CAD build for the part. Positions are in the model's coordinates, mm. Face numbers are marked on the shaded views. Round coordinates to 2 decimals unless told otherwise and drop trailing zeros. Order: outer loops, then holes, each group sorted by start corner. A loop starts at its lowest first (then second) coordinate and runs counter-clockwise, first axis right, second up. Notation, with made-up numbers: M 74.25,12 L 124.25,12 A26 cw 124.25,27 Z; hole C 29.5,67.5 d3. An arc over 180 degrees is marked long. Put each result on its own line as item: value.
```python
from build123d import *

# Parameters (mm, degrees)
SKETCH1_R           = 6
SKETCH1_R_2         = 3
BOSS_EXTRUDE1_DEPTH = 3
SKETCH3_R           = 3
BOSS_EXTRUDE3_DEPTH = 3
SKETCH4_R           = 8
SKETCH4_R_2         = 3
BOSS_EXTRUDE4_DEPTH = 12
SKETCH6_R           = 8
SKETCH6_R_2         = 3
BOSS_EXTRUDE5_DEPTH = 12


with BuildPart() as part:
    # Sketch1 → Boss-Extrude1 (new body)
    # profile 1 of 4: a face of its own
    with BuildSketch(Plane(origin=(0, 0, 0), x_dir=(1, 0, 0), z_dir=(0, 1, 0))):
        with BuildLine():
            ThreePointArc((42.894958583, -3.003752345), (43.557934635, -6.502479184), (45.856433127, -9.222319513))
            ThreePointArc((45.856433127, -9.222319513), (50.229473419, -29), (30.914979544, -35.101676259))
            ThreePointArc((30.914979544, -35.101676259), (27.410279478, -34.471038339), (24.048805129, -35.646247655))
            ThreePointArc((24.048805129, -35.646247655), (0, -43), (-24.048805129, -35.646247655))
            ThreePointArc((-24.048805129, -35.646247655), (-27.410279478, -34.471038339), (-30.914979544, -35.101676259))
            ThreePointArc((-30.914979544, -35.101676259), (-50.229473419, -29), (-45.856433127, -9.222319513))
            ThreePointArc((-45.856433127, -9.222319513), (-43.557934635, -6.502479184), (-42.894958583, -3.003752345))
            ThreePointArc((-42.894958583, -3.003752345), (-37.239092363, 21.5), (-18.846153454, 38.65))
            ThreePointArc((-18.846153454, 38.65), (-16.147655157, 40.973517523), (-14.941453584, 44.323995772))
            ThreePointArc((-14.941453584, 44.323995772), (0, 58), (14.941453584, 44.323995772))
            ThreePointArc((14.941453584, 44.323995772), (16.147655157, 40.973517523), (18.846153454, 38.65))
            ThreePointArc((18.846153454, 38.65), (37.239092363, 21.5), (42.894958583, -3.003752345))
        make_face()
        with Locations((37.239092363, -21.5)):
            Circle(SKETCH1_R, mode=Mode.SUBTRACT)
        with Locations((-37.239092363, -21.5)):
            Circle(SKETCH1_R, mode=Mode.SUBTRACT)
        with Locations((0, 43)):
            Circle(SKETCH1_R, mode=Mode.SUBTRACT)
    # profile 2 of 4: a face of its own
    with BuildSketch(Plane(origin=(0, 0, 0), x_dir=(1, 0, 0), z_dir=(0, 1, 0))):
        with Locations((-37.239092363, -21.5)):
            Circle(SKETCH1_R)
        with Locations(Location((-37.239092363, -21.5, 0), (0, 0, 270))):
            Circle(SKETCH1_R_2, mode=Mode.SUBTRACT)
    # profile 3 of 4: a face of its own
    with BuildSketch(Plane(origin=(0, 0, 0), x_dir=(1, 0, 0), z_dir=(0, 1, 0))):
        with Locations((37.239092363, -21.5)):
            Circle(SKETCH1_R)
        with Locations(Location((37.239092363, -21.5, 0), (0, 0, 270))):
            Circle(SKETCH1_R_2, mode=Mode.SUBTRACT)
    # profile 4 of 4: a face of its own
    with BuildSketch(Plane(origin=(0, 0, 0), x_dir=(1, 0, 0), z_dir=(0, 1, 0))):
        with Locations((0, 43)):
            Circle(SKETCH1_R)
        with Locations(Location((0, 43, 0), (0, 0, 270))):
            Circle(SKETCH1_R_2, mode=Mode.SUBTRACT)
    extrude(amount=BOSS_EXTRUDE1_DEPTH)

    # Sketch3 → Boss-Extrude3 (add)
    with BuildSketch(Plane(origin=(0, 3, 0), x_dir=(1, 0, 0), z_dir=(0, 1, 0))):
        with BuildLine():
            ThreePointArc((13.496951609, 40.286875), (0, 53.5), (-13.496951609, 40.286875))
            ThreePointArc((-13.496951609, 40.286875), (-14.175747319, 38.14126951), (-15.905498529, 36.701704545))
            ThreePointArc((-15.905498529, 36.701704545), (-34.641016151, 20), (-39.737357763, -4.576286487))
            ThreePointArc((-39.737357763, -4.576286487), (-40.119181988, -6.794077459), (-41.637932994, -8.454734533))
            ThreePointArc((-41.637932994, -8.454734533), (-46.332359102, -26.75), (-28.140981385, -31.832140467))
            ThreePointArc((-28.140981385, -31.832140467), (-25.943434669, -31.347192051), (-23.831859234, -32.125418059))
            ThreePointArc((-23.831859234, -32.125418059), (0, -40), (23.831859234, -32.125418059))
            ThreePointArc((23.831859234, -32.125418059), (25.943434669, -31.347192051), (28.140981385, -31.832140467))
            ThreePointArc((28.140981385, -31.832140467), (46.332359102, -26.75), (41.637932994, -8.454734533))
            ThreePointArc((41.637932994, -8.454734533), (40.119181988, -6.794077459), (39.737357763, -4.576286487))
            ThreePointArc((39.737357763, -4.576286487), (34.641016151, 20), (15.905498529, 36.701704545))
            ThreePointArc((15.905498529, 36.701704545), (14.175747319, 38.14126951), (13.496951609, 40.286875))
        make_face()
        with Locations(Location((0, 43, 0), (0, 0, 270))):
            Circle(SKETCH3_R, mode=Mode.SUBTRACT)
        with Locations(Location((-37.239092363, -21.5, 0), (0, 0, 270))):
            Circle(SKETCH3_R, mode=Mode.SUBTRACT)
        with Locations(Location((37.239092363, -21.5, 0), (0, 0, 270))):
            Circle(SKETCH3_R, mode=Mode.SUBTRACT)
    extrude(amount=BOSS_EXTRUDE3_DEPTH)

    # Sketch4 → Boss-Extrude4 (add)
    with BuildSketch(Plane(origin=(0, 6, 0), x_dir=(1, 0, 0), z_dir=(0, 1, 0))):
        with Locations(Location((0, 43, 0), (0, 0, 270))):
            Circle(SKETCH4_R)
        with Locations(Location((0, 43, 0), (0, 0, 270))):
            Circle(SKETCH4_R_2, mode=Mode.SUBTRACT)
    extrude(amount=BOSS_EXTRUDE4_DEPTH)

    # Sketch6 → Boss-Extrude5 (add)
    # profile 1 of 2: a face of its own
    with BuildSketch(Plane(origin=(0, 6, 0), x_dir=(1, 0, 0), z_dir=(0, 1, 0))):
        with Locations(Location((-37.239092363, -21.5, 0), (0, 0, 270))):
            Circle(SKETCH6_R)
        with Locations(Location((-37.239092363, -21.5, 0), (0, 0, 270))):
            Circle(SKETCH6_R_2, mode=Mode.SUBTRACT)
    # profile 2 of 2: a face of its own
    with BuildSketch(Plane(origin=(0, 6, 0), x_dir=(1, 0, 0), z_dir=(0, 1, 0))):
        with Locations(Location((37.239092363, -21.5, 0), (0, 0, 270))):
            Circle(SKETCH6_R)
        with Locations(Location((37.239092363, -21.5, 0), (0, 0, 270))):
            Circle(SKETCH6_R_2, mode=Mode.SUBTRACT)
    extrude(amount=BOSS_EXTRUDE5_DEPTH)


solid = part.part
```
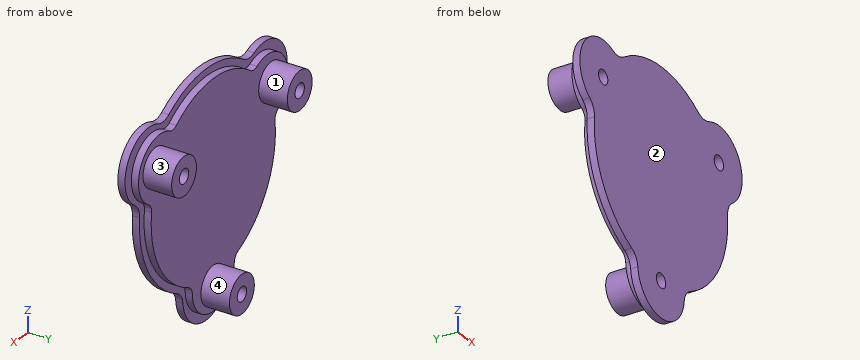
Item 1: Mould opens along X. For the marked faces 1, 2, 3 and 4 say: pulls with the +X half, pulls with the -X half, needs draft (parallel to the pull), parting line crosses it, or undercut.
Answers below:
face 1: undercut
face 2: needs draft
face 3: undercut
face 4: parting line crosses it
Item 2: Probe line 1 along X through (y, z) = (11, 21.5); line 2 along X through (y, z) = (12.75, -43); line 3 along X through (y, z) = (11.5, 19.5). List the from-to ranges inside material, lowest first. Write a range as [from, to].
Answers below:
line 1: [-45.24, -40.24], [-34.24, -29.24], [29.24, 34.24], [40.24, 45.24]
line 2: [-8, -3], [3, 8]
line 3: [-44.99, -39.48], [-35, -29.49], [29.49, 35], [39.48, 44.99]
Item 3: Pin check, flat tips, straight feed: P1, Ø10, axis at x = 36.5, y = 16, coming from the +Z side; P2, Ø12, axis at x = 15.5, z = -25, coming from the +Y side; P3, Ø8, axis at y = 6.5, z = -46.5, coming from the +X side; P4, Ø6, axis at x = 15, z = 25, coming from the -Y side. Stop position of each tip, or through.
Answers below:
P1: z = 29.5
P2: y = 6
P3: x = 14.92
P4: y = 0
Item 4: Band-saw the part on C-C on y = 13.5. Give the cut face in (x, z).
Answers below:
outline: C -37.24,21.5 d16; C 0,-43 d16; C 37.24,21.5 d16; hole C -37.24,21.5 d6; hole C 0,-43 d6; hole C 37.24,21.5 d6
Item 5: Band-saw the part on D-D on z = 20. Give the cut face in (x, y).
Answers below:
outline: M -52.16,0 L -39.84,0 L -39.84,18 L -45.1,18 L -45.1,6 L -48.14,6 L -48.14,3 L -52.16,3 Z; M -34.64,0 L 34.64,0 L 34.64,18 L 29.38,18 L 29.38,6 L -29.38,6 L -29.38,18 L -34.64,18 Z; M 39.84,0 L 52.16,0 L 52.16,3 L 48.14,3 L 48.14,6 L 45.1,6 L 45.1,18 L 39.84,18 Z
Item 6: Band-saw the part on A-A on x = 0. Give the cut face in (y, z).
Answers below:
outline: M 0,-58 L 3,-58 L 3,-53.5 L 6,-53.5 L 6,-51 L 18,-51 L 18,-46 L 0,-46 Z; M 0,-40 L 18,-40 L 18,-35 L 6,-35 L 6,40 L 3,40 L 3,43 L 0,43 Z
Item 7: Band-saw the part on B-B on z = -43. Give the cut face in (x, y).
Answers below:
outline: M -15.19,0 L -3,0 L -3,18 L -8,18 L -8,6 L -13.16,6 L -13.16,3 L -15.19,3 Z; M 3,0 L 15.19,0 L 15.19,3 L 13.16,3 L 13.16,6 L 8,6 L 8,18 L 3,18 Z
